For this review, take the finished solid that the model builds, in its own axes (mm). A direction names the side the tool comes from. Give positions to 0.01 mm unless a question says otherwise; leave off trailing zeros. Loops run counter-clockwise (first coordinate to the right, second up) from the corner with the lowest first, then second, coordinate; pieces in that order, holes last. Notation, with made-up numbers: (57, 38.25) -> (75, 38.25) arc R8 ccw to (75, 47.25) -> close; hole circle Ø1 at (13, 31.5). An arc over 180 degrees is marked (long way). Answer as CSV lines item,"result". Start each with the question number.
Item 1: Machinability: for faces 5 (the face through (-40.21, 17.4, -9.86)), 6 (the face through (-16, -18, 0)), 7 (the face through (-8.112, -19.524, -4.336)), which of the approach directions +Z, -Z, +X, -X, +Y, -Y give a long, thin tool a straight path to every point of the face, cutting with its end or side? Answer none if there is none.
Item 2: Clearance check with flat-ended pins moving along their axes: P1, Ø2, axis at x = -17.5, z = 1, coming from the +Y side; P2, Ø20, axis at y = -1, z = -0.5, coming from the -X side; P3, Ø10, axis at x = -10.5, z = -13, coming from the +Y side; P4, Ø1.5, axis at x = -6.5, y = -1, coming from the +Z side. State where each tip first meets the part, or that it passes through.
Item 3: Add section C-C on x = -29. State the section outline as (y, z) points.
Item 4: Add section A-A on y = 0. State the section outline as (x, z) points, plus the area to 3 significant figures.
Item 5: Add section B-B on x = -49. State the section outline as (y, z) points.
Item 6: The part is to be moulded in two halves that separate along X. For faces 1 (the face through (-40, 0, -20)), 2 (the face through (-25, -17, 5)), 3 (the face through (-20.56, 5.26, 16.69)), 4 (the face through (-18.269, 13.318, -1.749)), say which applies: +X half, -X half, draft (parallel to the pull), parting line (faces both ways), or undercut.
Item 7: For L1, parallel to Z at x = -46, y = 0; L2, parallel to Y at x = -42.5, z = 0; L3, parallel to X at y = -11.5, z = 15.5, list the stretches that pass through material, from the lowest coordinate up. Write a range as from..to.
```python
from build123d import *

# Parameters (mm, degrees)
F2_R     = 17.5
F3_DEPTH = 30
F4_R     = 11.75
F5_DEPTH = 55.001


with BuildPart() as f1:
    # F0 (on Front) → F1 (revolve)
    with BuildSketch(Plane.XZ):
        Polygon((-55, 17.5), (-55, 0), (-36.929604, 0), (-34, 11.75), (-30.240321, 11.75), (0, 16), (0, 20), (-16, 20), (-16, 17.5), align=None)
    revolve(axis=Axis((-27.5, 0, 0), (-1, 0, 0)))

    # F2 (on face) → F3 (join)
    with BuildSketch(Plane(origin=(-55, 0, 0), x_dir=(0, -1, 0), z_dir=(-1, 0, 0))):
        Polygon((11.547005, -20), (23.094011, 0), (11.547005, 20), (-11.547005, 20), (-23.094011, 0), (-11.547005, -20), align=None)
        Circle(F2_R, mode=Mode.SUBTRACT)
    extrude(amount=-F3_DEPTH)

    # F4 (on face) → F5 (cut, through all)
    with BuildSketch(Plane(origin=(-55, 0, 0), x_dir=(0, -1, 0), z_dir=(-1, 0, 0))):
        Circle(F4_R)
    extrude(amount=-F5_DEPTH, mode=Mode.SUBTRACT)


solid = f1.part
```
Computed values:
1,face 5,"-Z, +X, -X, +Y"
1,face 6,"none"
1,face 7,"+X"
2,P1,"y = 17.5"
2,P2,"through"
2,P3,"y = 18.33"
2,P4,"z = 20"
3,outline,"(-23.09, 0) -> (-11.55, -20) -> (11.55, -20) -> (23.09, 0) -> (11.55, 20) -> (-11.55, 20) -> close; hole circle Ø23.85 at (0, 0)"
4,outline,"(-55, -20) -> (-25, -20) -> (-25, -17.5) -> (-16, -17.5) -> (-16, -20) -> (0, -20) -> (0, -16) -> (-30.24, -11.75) -> (-55, -11.75) -> close; (-55, 11.75) -> (-30.24, 11.75) -> (0, 16) -> (0, 20) -> (-16, 20) -> (-16, 17.5) -> (-25, 17.5) -> (-25, 20) -> (-55, 20) -> close"
4,area,"734 mm²"
5,outline,"(-23.09, 0) -> (-11.55, -20) -> (11.55, -20) -> (23.09, 0) -> (11.55, 20) -> (-11.55, 20) -> close; hole circle Ø23.5 at (0, 0)"
6,face 1,"draft"
6,face 2,"undercut"
6,face 3,"undercut"
6,face 4,"+X half"
7,L1,"-20..-11.75, 11.75..20"
7,L2,"-23.09..-11.75, 11.75..23.09"
7,L3,"-55..-25, -16..0"
